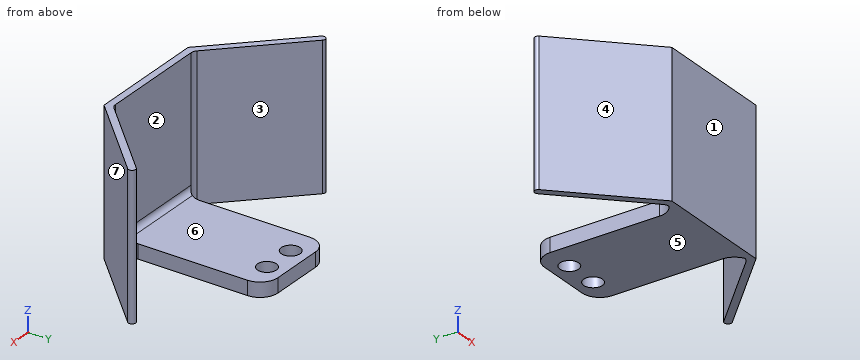
```python
from build123d import *

# Parameters (mm, degrees)
BOSS_EXTRUDE2_DEPTH = 40
FILLET1_R           = 4
SKETCH3_W           = 50
SKETCH3_H           = 8
BOSS_EXTRUDE3_DEPTH = 80
SKETCH5_R           = 5.25
CUT_EXTRUDE1_DEPTH  = 133.827565624
FILLET2_R           = 10
FILLET3_R           = 3


with BuildPart() as part:
    # Sketch2 → Boss-Extrude2 (new, symmetric)
    with BuildSketch(Plane.XY):
        with BuildLine():
            Line((-32, 0), (32, 0))
            Line((32, 0), (74.426406871, 42.426406871))
            ThreePointArc((74.426406871, 42.426406871), (77.254833996, 42.426406871), (77.254833996, 39.597979746))
            Line((77.254833996, 39.597979746), (33.656854249, -4))
            Line((33.656854249, -4), (-33.656854249, -4))
            Line((-33.656854249, -4), (-77.254833996, 39.597979746))
            ThreePointArc((-77.254833996, 39.597979746), (-77.254833996, 42.426406871), (-74.426406871, 42.426406871))
            Line((-74.426406871, 42.426406871), (-32, 0))
        make_face()
    extrude(amount=BOSS_EXTRUDE2_DEPTH, both=True)

    # Fillet1
    fillet1_edges = [part.edges().sort_by_distance(p)[0] for p in [
        (-32, 0, 0),
        (32, 0, 0),
    ]]
    fillet(fillet1_edges, radius=FILLET1_R)

    # Sketch3 → Boss-Extrude3 (add)
    with BuildSketch(Plane(origin=(0, 0, 0), x_dir=(1, 0, 0), z_dir=(0, 1, 0))):
        with Locations((0, 36)):
            Rectangle(SKETCH3_W, SKETCH3_H)
    extrude(amount=BOSS_EXTRUDE3_DEPTH)

    # Sketch5 → Cut-Extrude1 (cut, through all)
    with BuildSketch(Plane.XY.offset(-32)):
        with Locations((-9.5, 70)):
            Circle(SKETCH5_R)
        with Locations((9.5, 70)):
            Circle(SKETCH5_R)
    extrude(amount=-CUT_EXTRUDE1_DEPTH, mode=Mode.SUBTRACT)

    # Fillet2
    # the kernel refuses this fillet: 10 mm, written as the material it adds along each edge
    with BuildSketch(Plane(origin=(25, 0, -40), x_dir=(1, 0, 0), z_dir=(0, 0, 1)), Plane(origin=(-25, 0, -32), x_dir=(-1, 0, 0), z_dir=(0, 0, -1))) as fillet2_piece_1:
        with BuildLine():
            CenterArc((10, 8.849503291), FILLET2_R, 180, 62.245409403)
            Line((0, 8.849503291), (0, 0))
            Line((0, 0), (5.343145751, 0))
        make_face()
    extrude(amount=8)
    # the kernel refuses this fillet: 10 mm, written as the material it takes off along each edge
    with BuildSketch(Plane(origin=(25, 80, -65), x_dir=(-1, 0, 0), z_dir=(0, 0, 1))) as fillet2_2_piece_1:
        with BuildLine():
            CenterArc((FILLET2_R, FILLET2_R), FILLET2_R, 180, 90)
            Line((0, FILLET2_R), (0, 0))
            Line((0, 0), (FILLET2_R, 0))
        make_face()
    extrude(amount=58, mode=Mode.SUBTRACT)
    with BuildSketch(Plane(origin=(-25, 80, -7), x_dir=(0, -1, 0), z_dir=(0, 0, -1))) as fillet2_2_piece_2:
        with BuildLine():
            CenterArc((FILLET2_R, -FILLET2_R), FILLET2_R, 90, 90)
            Line((0, -FILLET2_R), (0, 0))
            Line((0, 0), (FILLET2_R, 0))
        make_face()
    extrude(amount=58, mode=Mode.SUBTRACT)

    # Fillet3
    # the kernel refuses this fillet: 3 mm, written as the material it adds along each edge
    with BuildSketch(Plane(origin=(-37.843145751, 0, -32), x_dir=(0, 1, 0), z_dir=(1, 0, 0))) as fillet3_piece_1_section:
        with BuildLine():
            CenterArc((FILLET3_R, FILLET3_R), FILLET3_R, 180, 90)
            Line((0, FILLET3_R), (0, 0))
            Line((0, 0), (FILLET3_R, 0))
        make_face()
    fillet3_piece_1 = extrude(amount=75.686291501, mode=Mode.PRIVATE)
    fillet3_piece_1 = fillet3_piece_1 - Plane(origin=(35, 8.849503291, -32), x_dir=(1, 0, 0), z_dir=(0, 0, -1)) * Cylinder(10, 164, mode=Mode.PRIVATE)
    fillet3_piece_1 = fillet3_piece_1 - Plane(origin=(-35, 8.849503291, -32), x_dir=(-1, 0, 0), z_dir=(0, 0, 1)) * Cylinder(10, 164, mode=Mode.PRIVATE)
    add(fillet3_piece_1)


solid = part.part
```
Read the model definition and answer for the solid it produces. Units are mm, in the model's axes. Face numbers are marked on the shaded views. A direction names the side the tool comes from. Coordinates: 2 decimals unless noted, no trailing zeros. Order: outer loops, then holes, each group sorted by start corner. A loop starts at its lowest first (then second) coordinate and runs counter-clockwise, first axis right, second up. Notation, with made-up numbers: (48, 24) - (77, 24) arc R17 cw to (77, 43) - close; hole circle Ø5 at (38.25, 34). An arc over 180 degrees is marked (long way). Answer as a JSON object with one key per item and string values. Group by question number.
Item 1: The mould has two halves that part along X. Classify the marked faces 4, 5, 6 and 7: +X half, -X half, draft (parallel to the pull), parting line (faces both ways), or undercut.
Item 2: Section A-A (x = -9.5) is taken. Give the vertices of the cut face in (y, z).
Item 3: A tool of negligible diameter and unlimited length cuts with its end or side. For the marked faces 1, 2 and 3, from which of +Z, -Z, +X, -X, +Y, -Y can it reach the whole face along a straight path? Write none if from no direction.
Item 4: Flat-ended cylindrical pins translate along their axes: P1, Ø13.5, axis at x = -9.5, y = 70, coming from the +Z side; P2, Ø12, axis at x = -52, z = -30, coming from the -Y side; P3, Ø2.5, axis at y = 48.5, z = -36.5, coming from the -X side. Find the tip coordinate at first contact, or state that the pin passes through.
Item 5: Consider probe 1 along Y at (x, z) = (-9.5, -34); probe 2 along Z at (x, y) = (13, 42); probe 3 along Y at (x, z) = (23, 5.5). Determine where each line is inside the solid, lowest interval first. Write a range as from..to.
Item 6: Section D-D (x = 35.5) is taken. Give the vertices of the cut face in (y, z), plus the area to 3 significant figures.
Item 7: Section B-B (z = 14.5) is taken. Give the vertices of the cut face in (x, y), plus the area to 3 significant figures.
Item 8: Section C-C (y = 35) is taken. Give the vertices of the cut face in (x, z).
Results are:
{
 "1": {"face 4": "-X half", "face 5": "draft", "face 6": "undercut", "face 7": "+X half"},
 "2": {"outline": "(-4, -40) - (64.75, -40) - (64.75, -32) - (3, -32) arc R3 cw to (0, -29) - (0, 40) - (-4, 40) - close; (75.25, -40) - (80, -40) - (80, -32) - (75.25, -32) - close"},
 "3": {"face 1": "+Z, -Z, +X, -X, -Y", "face 2": "+Z, +Y", "face 3": "+Z, -Z, +Y"},
 "4": {"P1": "stops at z = -32", "P2": "stops at y = 8.34", "P3": "stops at x = -25"},
 "5": {"probe 1": "y = -4..64.75, 75.25..80", "probe 2": "z = -40..-32", "probe 3": "y = -4..0"},
 "6": {"outline": "(-2.16, -40) - (3.5, -40) - (3.5, 40) - (-2.16, 40) - close", "area": "453 mm^2"},
 "7": {"outline": "(-77.25, 39.6) - (-33.66, -4) - (33.66, -4) - (77.25, 39.6) arc R2 ccw to (74.43, 42.43) - (33.17, 1.17) arc R4 cw to (30.34, 0) - (-30.34, 0) arc R4 cw to (-33.17, 1.17) - (-74.43, 42.43) arc R2 ccw to start", "area": "763 mm^2"},
 "8": {"outline": "(-72.66, -40) - (-67, -40) - (-67, 40) - (-72.66, 40) - close; (-25, -40) - (25, -40) - (25, -32) - (-25, -32) - close; (67, -40) - (72.66, -40) - (72.66, 40) - (67, 40) - close"}
}
